The listing builds one solid part. Answer for the finished solid, in the listing's coordinates (mm). Round coordinates to 2 decimals unless told otherwise and drop trailing zeros. Loops run counter-clockwise (first coordinate to the right, second up) from the corner with the lowest first, then second, coordinate; pieces in that order, holes last. Notation, with made-up numbers: M 65.5,22 L 98.5,22 A6 ccw 98.5,31 Z; hole C -28,30.25 d4. An arc over 180 degrees is marked long. Put each result on its own line as item: value. Start each with the question number.
(1) Flat-ended cylindrical pins translate along their axes: P1, Ø12, axis at x = 7.5, y = -56, coming from the -Z side; P2, Ø5, axis at x = -7.5, y = -3.5, coming from the -Z side; P3, Ø5, axis at x = 0, z = 0, coming from the +Y side. Find the tip coordinate at first contact, or state that the pin passes through.
(2) Straight lines are drawn through the part: line 1 (X direction, y = 127.25, z = 0); line 2 (X direction, y = -66.5, z = -1). For each, find the intervals that lie inside material, in ascending order.
(3) Section A-A, the plane y = 11 is taken. Determine the outline of the cut face in (x, z).
```python
from build123d import *

# Parameters (mm, degrees)
SKETCH1_W     = 10
SKETCH1_H     = 265
CHAMFER1_SIZE = 1


with BuildPart() as part:
    # Sketch1 → Revolve2 (revolve)
    with BuildSketch(Plane.XY):
        with Locations((-5, 0)):
            Rectangle(SKETCH1_W, SKETCH1_H)
    revolve(axis=Axis((0, 132.5, 0), (0, -1, 0)))

    # Sketch3 → M10 Tapped Hole1 (revolve, cut)
    with BuildSketch(Plane(origin=(0, -132.5, 0), x_dir=(0, 0, -1), z_dir=(1, 0, 0))):
        Polygon((0, 0), (0, 27.053657631), (4.25, 24.5), (4.25, 0), align=None)
    m10_tapped_hole1 = revolve(axis=Axis((0, -138.85, 0), (0, 1, 0)), mode=Mode.SUBTRACT)

    # Mirror1: M10 Tapped Hole1 across plane
    add(m10_tapped_hole1.mirror(Plane.ZX), mode=Mode.SUBTRACT)

    # Chamfer1
    chamfer1_edges = [part.edges().sort_by_distance(p)[0] for p in [
        (10, -132.5, 0),
        (10, 132.5, 0),
    ]]
    chamfer(chamfer1_edges, length=CHAMFER1_SIZE)


solid = part.part
```
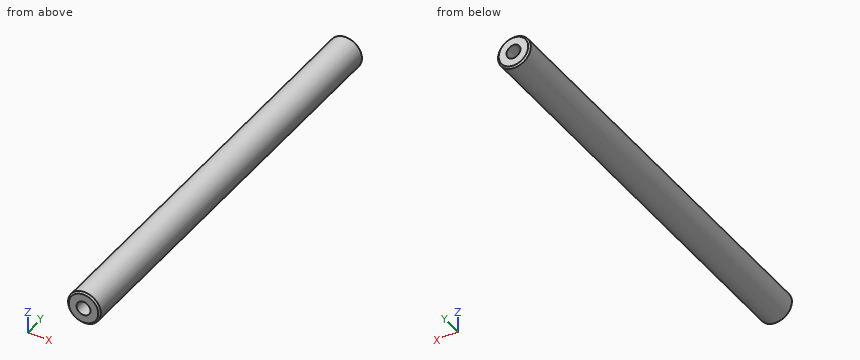
Recorded:
1. P1: stops at z = -9.89
1. P2: stops at z = -8.66
1. P3: stops at y = 106.95
2. line 1: x = -10 to -4.25, 4.25 to 10
2. line 2: x = -9.95 to 9.95
3. outline: C 0,0 d20
